Check sheet for the modelled part. Datum: model origin and axes. Units: mm. A direction names the side the tool comes from. Coordinates: 2 decimals unless noted, no trailing zeros. Loops run counter-clockwise (first coordinate to the right, second up) from the corner with the lowest first, then second, coordinate; pieces in that order, holes last. Notation, with made-up numbers: M 88.5,72.5 L 133.5,72.5 A26 ccw 133.5,89.5 Z; hole C 5,69.25 d11. An arc over 180 degrees is marked long. Answer in a Markdown table with one row per item. Add a question column.
```python
from build123d import *

# Parameters (mm, degrees)
BOSS_EXTRUDE1_START        = 0.2
SKETCH2_R                  = 4.05
BOSS_EXTRUDE1_DEPTH        = 0.2
BOSS_EXTRUDE1_DEPTH_BACK   = 3
BOSS_EXTRUDE1_2_DEPTH      = 0.2
BOSS_EXTRUDE1_2_DEPTH_BACK = 3
BOSS_EXTRUDE2_START        = 0.4
SKETCH2_8_R                = 2.95
BOSS_EXTRUDE2_DEPTH        = 2
BOSS_EXTRUDE3_START        = 0.4
SKETCH2_10_R               = 2.95
BOSS_EXTRUDE3_DEPTH        = 5.9
BOSS_EXTRUDE4_START        = -5.5
SKETCH2_11_R               = 2.95
SKETCH2_11_R_2             = 1.55
BOSS_EXTRUDE4_DEPTH        = 4.3
BOSS_EXTRUDE5_DEPTH        = 1.3


with BuildPart() as part:
    # Sketch2 → Boss-Extrude1 (new body, two sides)
    with BuildSketch(Plane.XZ.offset(17.641705272).offset(BOSS_EXTRUDE1_START)) as boss_extrude1_sk:
        with Locations((41.993031242, -65.814080244)):
            Circle(SKETCH2_R)
    extrude(amount=BOSS_EXTRUDE1_DEPTH)
    extrude(boss_extrude1_sk.sketch, amount=-BOSS_EXTRUDE1_DEPTH_BACK)



with BuildPart() as body_2:
    # Sketch2 → Boss-Extrude1 2 (new body, two sides)
    with BuildSketch(Plane.XZ.offset(17.641705272).offset(BOSS_EXTRUDE1_START)) as boss_extrude1_2_sk:
        with Locations((63.743031242, -65.814080244)):
            Circle(SKETCH2_R)
    extrude(amount=BOSS_EXTRUDE1_2_DEPTH)
    extrude(boss_extrude1_2_sk.sketch, amount=-BOSS_EXTRUDE1_2_DEPTH_BACK)


with BuildPart() as part_1:
    add(part.part)

    add(body_2.part)  # Boss-Extrude2 merges body 2
    # Sketch2_8 → Boss-Extrude2 (add)
    with BuildSketch(Plane.XZ.offset(17.641705272).offset(BOSS_EXTRUDE2_START)):
        with BuildLine():
            Line((43.332476509, -57.294092988), (62.403585975, -57.294092988))
            ThreePointArc((62.403585975, -57.294092988), (65.403585975, -58.097940565), (67.599738397, -60.294092988))
            Line((67.599738397, -60.294092988), (69.025786205, -62.764080244))
            ThreePointArc((69.025786205, -62.764080244), (69.025786205, -68.864080244), (63.743031242, -71.914080244))
            Line((63.743031242, -71.914080244), (41.993031242, -71.914080244))
            ThreePointArc((41.993031242, -71.914080244), (36.710276279, -68.864080244), (36.710276279, -62.764080244))
            Line((36.710276279, -62.764080244), (38.136324086, -60.294092988))
            ThreePointArc((38.136324086, -60.294092988), (40.332476509, -58.097940565), (43.332476509, -57.294092988))
        make_face()
        with Locations((52.868031242, -61.584989522)):
            Circle(SKETCH2_8_R, mode=Mode.SUBTRACT)
    extrude(amount=BOSS_EXTRUDE2_DEPTH)

    # Sketch2_10 → Boss-Extrude3 (add)
    with BuildSketch(Plane.XZ.offset(17.641705272).offset(BOSS_EXTRUDE3_START)):
        with BuildLine():
            Line((53.128785981, -57.294092988), (52.607276503, -57.294092988))
            ThreePointArc((52.607276503, -57.294092988), (48.904424631, -59.236968036), (48.39898543, -63.387920534))
            ThreePointArc((48.39898543, -63.387920534), (48.681708279, -67.291950162), (46.7804094, -70.713417992))
            ThreePointArc((46.7804094, -70.713417992), (46.621377652, -71.478216974), (47.269630525, -71.914080244))
            Line((47.269630525, -71.914080244), (58.466431958, -71.914080244))
            ThreePointArc((58.466431958, -71.914080244), (59.114684832, -71.478216974), (58.955653084, -70.713417992))
            ThreePointArc((58.955653084, -70.713417992), (57.054354205, -67.291950162), (57.337077053, -63.387920534))
            ThreePointArc((57.337077053, -63.387920534), (56.831637852, -59.236968036), (53.128785981, -57.294092988))
        make_face()
        with Locations((52.868031242, -61.584989522)):
            Circle(SKETCH2_10_R, mode=Mode.SUBTRACT)
    extrude(amount=-BOSS_EXTRUDE3_DEPTH)

    # Sketch2_11 → Boss-Extrude4 (add)
    with BuildSketch(Plane.XZ.offset(17.641705272).offset(BOSS_EXTRUDE4_START)):
        with Locations((52.868031242, -61.584989522)):
            Circle(SKETCH2_11_R)
        with Locations((52.868031242, -61.584989522)):
            Circle(SKETCH2_11_R_2, mode=Mode.SUBTRACT)
    extrude(amount=BOSS_EXTRUDE4_DEPTH)

    # Sketch3 → Boss-Extrude5 (add)
    with BuildSketch(Plane(origin=(0, -12.141705272, 0), x_dir=(1, 0, 0), z_dir=(0, 1, 0))):
        Polygon((50.091896525, 70.773300161), (52.868031242, 67.410555891), (55.644165958, 70.773300161), (56.83946806, 69.786510981), (54.182101398, 66.567630982), (55.859200009, 64.536154012), (54.663897908, 63.549364832), (52.868031242, 65.724706073), (51.072164576, 63.549364832), (49.876862474, 64.536154012), (51.553961085, 66.567630982), (48.896594423, 69.786510981), align=None)
    extrude(amount=BOSS_EXTRUDE5_DEPTH)


solid = part_1.part
```
Q1. Mould release check, pull along Z, two halves, no side actions. Record for faces 1 (the face through (52.666, -14.262, -60.048)), 2 (the face through (56.23, -11.5, -70.29)), 3 (the face through (64, -14.842, -66)): released by +Z, released by -Z, zero draft, split by the parting line, or undercut.
Q2. Thickness scan on L1, parallel to Y at x = 41.5, z = -59.25; L2, parallel to Y at x = 44.5, z = -64.25; L3, parallel to X at y = -18.25, z = -60.25. Record the ranges inside material, lowest first.
Q3. Access from +Z, -Z, +X, -X, +Y, -Y to the whole of each face (thin tool, end or side, straight path). Record for faces 4 (the face through (56.87, -15.13, -59.29)), 5 (the face through (50.48, -11.5, -64.04)), 6 (the face through (54.24, -11.5, -69.07)), 7 (the face through (55.27, -11.5, -64.05)), 8 (the face through (59.11, -15.13, -71.49)).
Q4. Cross-section at D-D (y = -14.5). Record the cut outline in (x, z).
Q5. Go/stop test with flat-tipped pins: pin 1 (4.5 mm diameter, centred on x = 52.87, z = -61.58, fed in from -Y); pin 2 (4 mm diameter, centred on x = 60, y = -17, fed in from +Z); pin 3 (3 mm diameter, centred on x = 64.5, z = -67.5, fed in from +Y); pin 4 (2 mm diameter, centred on y = -19, z = -60.5, fed in from -X). Record where each tip stops, or that it passes through.
Q6. Cross-section at A-A (y = -16). Record the cut outline in (x, z), plus the area to 3 significant figures.
Q7. Cross-section at B-B (z = -60.75). Record the cut outline in (x, y).
Q8. Cross-section at C-C (x = 60). Record the cut outline in (y, z), plus the area to 3 significant figures.
Answer key:
| question | item | result |
|---|---|---|
| 1 | face 1 | undercut |
| 1 | face 2 | released by -Z |
| 1 | face 3 | zero draft |
| 2 | L1 | -20.04 to -18.04 |
| 2 | L2 | -20.04 to -14.84 |
| 2 | L3 | 38.16 to 50.24, 55.5 to 67.57 |
| 3 | face 4 | +Y |
| 3 | face 5 | +Z, -X, +Y |
| 3 | face 6 | -Z, +Y |
| 3 | face 7 | +Z, +X, +Y |
| 3 | face 8 | +X, +Y |
| 4 | outline | M 46.78,-70.71 A0.7 ccw 47.27,-71.91 L 58.47,-71.91 A0.7 ccw 58.96,-70.71 A6.85 cw 57.34,-63.39 A4.5 ccw 53.13,-57.29 L 52.61,-57.29 A4.5 ccw 48.4,-63.39 A6.85 cw Z; hole C 52.87,-61.58 d3.1 |
| 5 | pin 1 | y = -16.44 |
| 5 | pin 2 | z = -57.29 |
| 5 | pin 3 | y = -14.84 |
| 5 | pin 4 | x = 37.44 |
| 6 | outline | C 41.99,-65.81 d8.1; M 46.78,-70.71 A0.7 ccw 47.27,-71.91 L 58.47,-71.91 A0.7 ccw 58.96,-70.71 A6.85 cw 57.34,-63.39 A4.5 ccw 53.13,-57.29 L 52.61,-57.29 A4.5 ccw 48.4,-63.39 A6.85 cw Z; C 63.74,-65.81 d8.1; hole C 52.87,-61.58 d3.1 |
| 6 | area | 225 mm^2 |
| 7 | outline | M 37.87,-20.04 L 50.04,-20.04 L 50.04,-16.44 L 51.56,-16.44 L 51.56,-12.14 L 48.23,-12.14 L 48.23,-18.04 L 37.87,-18.04 Z; M 54.17,-16.44 L 55.7,-16.44 L 55.7,-20.04 L 67.86,-20.04 L 67.86,-18.04 L 57.51,-18.04 L 57.51,-12.14 L 54.17,-12.14 Z |
| 8 | outline | M -20.04,-71.91 L -18.04,-71.91 L -18.04,-67.36 L -14.84,-67.36 L -14.84,-64.27 L -18.04,-64.27 L -18.04,-57.29 L -20.04,-57.29 Z |
| 8 | area | 39.1 mm^2 |
